Input: part model. Units: mm. Frame: model coordinates. A direction names the side the tool comes from. Round coordinates to 2 decimals unless told otherwise and drop trailing zeros. Loops run counter-clockwise (first coordinate to the right, second up) from the corner with the lowest first, then second, coordinate; pieces in that order, holes last. Notation, with made-up numbers: (19, -16.5) -> (51, -16.5) arc R12 ccw to (51, 3.5) -> close; hole circle Ø1 at (-30, 31.25). An arc over 180 degrees is marked (long way). Answer as a JSON object with one key per item and string values.
```python
from build123d import *

# Parameters (mm, degrees)
SKETCH1_W           = 20
SKETCH1_H           = 20
SKETCH1_R           = 2.6
BOSS_EXTRUDE2_DEPTH = 3
SKETCH2_W           = 20
SKETCH2_H           = 3
BOSS_EXTRUDE3_DEPTH = 10
SKETCH4_R           = 2.6
CUT_EXTRUDE1_DEPTH  = 10
SKETCH6_W           = 20
SKETCH6_H           = 3
BOSS_EXTRUDE5_DEPTH = 5
SKETCH7_W           = 20
SKETCH7_H           = 5
BOSS_EXTRUDE6_DEPTH = 50
CUT_EXTRUDE2_DEPTH  = 5


with BuildPart() as part:
    # Sketch1 → Boss-Extrude2 (new body)
    with BuildSketch(Plane(origin=(0, 0, 0), x_dir=(1, 0, 0), z_dir=(0, 1, 0))):
        Rectangle(SKETCH1_W, SKETCH1_H)
        with Locations(Location((0, 0, 0), (0, 0, 270))):
            Circle(SKETCH1_R, mode=Mode.SUBTRACT)
    extrude(amount=BOSS_EXTRUDE2_DEPTH)

    # Sketch2 → Boss-Extrude3 (add)
    with BuildSketch(Plane.XY.offset(10)):
        with Locations((0, 1.5)):
            Rectangle(SKETCH2_W, SKETCH2_H)
    extrude(amount=BOSS_EXTRUDE3_DEPTH)

    # Sketch4 → Cut-Extrude1 (cut)
    with BuildSketch(Plane(origin=(0, 3, 0), x_dir=(1, 0, 0), z_dir=(0, 1, 0))):
        with Locations(Location((0, -15, 0), (0, 0, 270))):
            Circle(SKETCH4_R)
    extrude(amount=-CUT_EXTRUDE1_DEPTH, mode=Mode.SUBTRACT)

    # Sketch6 → Boss-Extrude5 (add)
    with BuildSketch(Plane(origin=(0, 0, -10), x_dir=(-1, 0, 0), z_dir=(0, 0, -1))):
        with Locations((0, 1.5)):
            Rectangle(SKETCH6_W, SKETCH6_H)
    extrude(amount=BOSS_EXTRUDE5_DEPTH)

    # Sketch7 → Boss-Extrude6 (add)
    with BuildSketch(Plane.XZ):
        with Locations((0, -12.5)):
            Rectangle(SKETCH7_W, SKETCH7_H)
    extrude(amount=BOSS_EXTRUDE6_DEPTH)

    # Sketch8 → Cut-Extrude2 (cut)
    with BuildSketch(Plane(origin=(0, 0, -15), x_dir=(-1, 0, 0), z_dir=(0, 0, -1))):
        with BuildLine():
            Line((-2.6, -25), (-2.6, -43))
            ThreePointArc((-2.6, -43), (0, -45.6), (2.6, -43))
            Line((2.6, -43), (2.6, -25))
            ThreePointArc((2.6, -25), (0, -22.4), (-2.6, -25))
        make_face()
    extrude(amount=-CUT_EXTRUDE2_DEPTH, mode=Mode.SUBTRACT)


solid = part.part
```
1) Ray query, probe 1 along X at (y, z) = (0.9, 0); probe 2 along Z at (x, y) = (-8.5, -35.5); probe 3 along Y at (x, z) = (-1.75, 5). Return the intervals inside material, ascending.
Output:
{"probe 1": "x = -10 to -2.6, 2.6 to 10", "probe 2": "z = -15 to -10", "probe 3": "y = 0 to 3"}
2) Section B-B, the plane x = 0. Output: boundary loops of the cut face in (y, z).
Output:
{"outline": "(-50, -15) -> (-45.6, -15) -> (-45.6, -10) -> (-50, -10) -> close; (-22.4, -15) -> (3, -15) -> (3, -2.6) -> (0, -2.6) -> (0, -10) -> (-22.4, -10) -> close; (0, 2.6) -> (3, 2.6) -> (3, 12.4) -> (0, 12.4) -> close; (0, 17.6) -> (3, 17.6) -> (3, 20) -> (0, 20) -> close"}
3) Reachability of faces 5 (the face through (0.1, -45.6, -12.5)), 6 (the face through (-10, -17, -11)) from +Z, -Z, +X, -X, +Y, -Y: full face, straight path, thin tool, end or side. Return the list, or none.
Output:
{"face 5": "+Z, -Z", "face 6": "+Z, -Z, -X, +Y, -Y"}
4) Section D-D, the plane z = 15. Output: boundary loops of the cut face in (x, y).
Output:
{"outline": "(-10, 0) -> (-2.6, 0) -> (-2.6, 3) -> (-10, 3) -> close; (2.6, 0) -> (10, 0) -> (10, 3) -> (2.6, 3) -> close"}
5) Section A-A, the plane z = -1. Output: boundary loops of the cut face in (x, y), plus the area to 3 significant figures.
Output:
{"outline": "(-10, 0) -> (-2.4, 0) -> (-2.4, 3) -> (-10, 3) -> close; (2.4, 0) -> (10, 0) -> (10, 3) -> (2.4, 3) -> close", "area": "45.6 mm^2"}
6) Draft query along Y for faces 1 (the face through (0, -19, -10)), 2 (the face through (2.6, -34, -13)), 3 (the face through (0, 0, 5)), 4 (the face through (-0.1, -22.4, -12.5)). Return one class per face: +Y half, -Y half, draft (parallel to the pull), parting line (faces both ways), or undercut.
Output:
{"face 1": "draft", "face 2": "undercut", "face 3": "-Y half", "face 4": "undercut"}
7) Contact query for flat-ended pins moving along their axis: P1, Ø10, axis at x = -3.5, y = -31.5, coming from the +Z side; P2, Ø6, axis at x = -7.5, z = 7, coming from the -Y side; P3, Ø5, axis at x = -0.5, y = -41.5, coming from the -Z side. Output: stop coordinate, or through.
Output:
{"P1": "stops at z = -10", "P2": "stops at y = 0", "P3": "stops at z = -15"}
8) Section C-C, the plane x = 7. Output: boundary loops of the cut face in (y, z), plus the area to 3 significant figures.
Output:
{"outline": "(-50, -15) -> (3, -15) -> (3, 20) -> (0, 20) -> (0, -10) -> (-50, -10) -> close", "area": "355 mm^2"}
